Read the model definition and answer for the solid it produces. Units are mm, in the model's axes. A direction names the side the tool comes from. Coordinates: 2 decimals unless noted, no trailing zeros. Write each loop counter-clockwise with the first axis right and the second up, starting at its lowest first coordinate (ties: lowest second). Pieces come first, ordered by that corner, then holes.
1) The part is cut by section A-A (y = 7). Determine the outline of the cut face in (x, z), then the cut area to 3 significant figures.
2) Determine the mould class of faces 4 (the face through (-1, -17.236, 3)), 5 (the face through (-20.363, -2, 3)), 6 (the face through (-2, 32.764, 3)), 7 (the face through (23.637, 8, 3)) for opening direction Y: +Y half, -Y half, draft (parallel to the pull), parting line (faces both ways), or undercut.
3) Which of the six approach directions +Z, -Z, +X, -X, +Y, -Y give full straight-line access (tool end or side, diameter ignored) to faces 1 (the face through (-26.363, -12, 3)), 2 (the face through (-20.363, 18, 3)), 3 (the face through (13.637, 25, 3))?
4) This flat-tipped pin is pushed along its axis until it touches: pin 1 Ø1.8 at (y, z) = (18, 1.5) entering from -X. Where does it stop, or does it pass through?
5) Find the intervals of material crossed by line 1 (Y direction, x = 13, z = 5.1); line 2 (Y direction, x = -21, z = 0.7); line 3 (X direction, y = -8, z = 1.4), in increasing order.
6) The part is cut by section D-D (z = 2). Determine the outline of the cut face in (x, y), then the cut area to 3 significant figures.
7) The part is cut by section B-B (x = -22.5). Determine the outline of the cut face in (y, z).
8) The part is cut by section C-C (x = 6.5). Determine the outline of the cut face in (y, z), then the cut area to 3 significant figures.
from build123d import *

# Parameters (mm, degrees)
SKETCH_1_W      = 10
SKETCH_1_H      = 6
EXTRUDE_1_DEPTH = 6


with BuildPart() as part:
    # 草圖1 → 填料-伸長1 (new body)
    with BuildSketch(Plane.XY):
        Polygon((-26.362898543, 32.763671875), (23.637101457, 32.763671875), (23.637101457, -17.236328125), (-26.362898543, -17.236328125), (-26.362898543, -7.236328125), (-20.362898543, -7.236328125), (-20.362898543, 2.763671875), (-26.362898543, 2.763671875), (-26.362898543, 12.763671875), (-20.362898543, 12.763671875), (-20.362898543, 22.763671875), (-26.362898543, 22.763671875), align=None)
        with Locations((8.637101457, 7.763671875)):
            Rectangle(SKETCH_1_W, SKETCH_1_H, mode=Mode.SUBTRACT)
        with Locations((8.637101457, 24.763671875)):
            Rectangle(SKETCH_1_W, SKETCH_1_H, mode=Mode.SUBTRACT)
        with Locations((8.637101457, -9.236328125)):
            Rectangle(SKETCH_1_W, SKETCH_1_H, mode=Mode.SUBTRACT)
    extrude(amount=EXTRUDE_1_DEPTH)


solid = part.part
Reported:
1. outline: (-26.36, 0) - (3.64, 0) - (3.64, 6) - (-26.36, 6) - close; (13.64, 0) - (23.64, 0) - (23.64, 6) - (13.64, 6) - close
1. area: 240 mm2
2. face 4: -Y half
2. face 5: undercut
2. face 6: +Y half
2. face 7: draft
3. face 1: +Z, -Z, -X, +Y, -Y
3. face 2: +Z, -Z, -X
3. face 3: +Z, -Z
4. pin 1: stops at x = -20.36
5. line 1: y = -17.24 to -12.24, -6.24 to 4.76, 10.76 to 21.76, 27.76 to 32.76
5. line 2: y = -17.24 to -7.24, 2.76 to 12.76, 22.76 to 32.76
5. line 3: x = -26.36 to 3.64, 13.64 to 23.64
6. outline: (-26.36, -17.24) - (23.64, -17.24) - (23.64, 32.76) - (-26.36, 32.76) - (-26.36, 22.76) - (-20.36, 22.76) - (-20.36, 12.76) - (-26.36, 12.76) - (-26.36, 2.76) - (-20.36, 2.76) - (-20.36, -7.24) - (-26.36, -7.24) - close; hole (3.64, -12.24) - (13.64, -12.24) - (13.64, -6.24) - (3.64, -6.24) - close; hole (3.64, 4.76) - (13.64, 4.76) - (13.64, 10.76) - (3.64, 10.76) - close; hole (3.64, 21.76) - (13.64, 21.76) - (13.64, 27.76) - (3.64, 27.76) - close
6. area: 2,200 mm2
7. outline: (-17.24, 0) - (-7.24, 0) - (-7.24, 6) - (-17.24, 6) - close; (2.76, 0) - (12.76, 0) - (12.76, 6) - (2.76, 6) - close; (22.76, 0) - (32.76, 0) - (32.76, 6) - (22.76, 6) - close
8. outline: (-17.24, 0) - (-12.24, 0) - (-12.24, 6) - (-17.24, 6) - close; (-6.24, 0) - (4.76, 0) - (4.76, 6) - (-6.24, 6) - close; (10.76, 0) - (21.76, 0) - (21.76, 6) - (10.76, 6) - close; (27.76, 0) - (32.76, 0) - (32.76, 6) - (27.76, 6) - close
8. area: 192 mm2
